Autodesk Inventor part; units mm, degrees
ref_plane "YZ Plane" through (0, 0, 0) normal (1, 0, 0) x (0, 1, 0)
ref_plane "XZ Plane" through (0, 0, 0) normal (0, 1, 0) x (-1, 0, 0)
ref_plane "XY Plane" through (0, 0, 0) normal (0, 0, 1) x (1, 0, 0)
sketch "Sketch1" plane through (0, 0, 0) normal (0, 0, 1) x (1, 0, 0)
  line L0 (0, 0) -> (-9.5, 0)
  line L1 (-9.5, 0) -> (-9.5, 110)
  line L2 (-9.5, 110) -> (-5.5705, 200)
  line L3 (-5.5705, 200) -> (-9, 228)
  line L4 (-9, 228) -> (-9, 232)
  line L5 (-9, 232) -> (-5, 232)
  line L6 (-5, 232) -> (-5, 235)
  line L7 (-5, 235) -> (-6, 235.5774)
  line L8 (-6, 235.5774) -> (-6, 250)
  line L9 (-6, 250) -> (0, 250)
  line L10 (0, 250) -> (0, 0)
  line L11 (0, -50) -> (0, 300)
  line L12 (-11.4, 0) -> (1.9, 0)
  dimension "d0" = 250
  dimension "d1" = 19
  dimension "d2" = 110
  dimension "d5" = 11.141
  dimension "d6" = 12
  dimension "d7" = 3
  dimension "d9" = 18
  dimension "d10" = 4
  dimension "d11" = 10
  dimension "d12" = 60
  dimension "d13" = 18
  dimension "d14" = 2.5
  dimension "d16" = 6.983
  dimension "d17" = 200
  dimension "d18" = 232
  dimension "d19" = 50
  dimension "d20" = 14.4227
revolve "Revolution1" add sketch "Sketch1" angle 360 about axis through (0, -10, 0) along (0, 1, 0)
thread "Thread1"
sketch "Sketch2" plane through (0, 0, 0) normal (0, -1, 0) x (1, 0, 0)
  circle A0 centre (0, 0) radius 9.5
hole "Hole1" at (0, 0, 0) direction (0, 1, 0) diameter 15 depth 80 tip angle 118
chamfer "Chamfer2" distance 2 angle 45 1 edges at (6, 250, 0)
chamfer "Chamfer3" distance 0.5 angle 45 1 edges at (0, 0, 7.5)
chamfer "Chamfer4" distance 1 angle 45 1 edges at (9.5, 0, 0)
properties part number "HM1-001" material "Steel, Alloy"
Part model, mm, in its own coordinate system. A direction names the side the tool comes from. Give positions to 0.01 mm unless a question says otherwise; leave off trailing zeros. Loops run counter-clockwise (first coordinate to the right, second up) from the corner with the lowest first, then second, coordinate; pieces in that order, holes last. Notation, with made-up numbers: (82, -11) -> (89, -11) arc R9 cw to (89, -1) -> close; hole circle Ø5 at (50.5, 19.5). An arc over 180 degrees is marked (long way). Write each question's results on one line, items separated by ' | '. Start each with the question number.
Q1. Band-saw the part on A-A on y = 97. List the corners of the cut face in (x, z).
Q2. Pin check, flat tips, straight feed: P1, Ø1, axis at y = 77.5, z = 6.5, coming from the -X side; P2, Ø6, axis at y = 41.5, z = 5.5, coming from the -X side; P3, Ø8, axis at y = 100, z = 2.5, coming from the +X side; P4, Ø6, axis at y = 142.5, z = -5, coming from the +X side. Stop position of each tip, or through.
Q3. Pull direction Y, two halves, no side cores. Call faces 1 (the face through (1.585, 214.196, -7.135)), 2 (the face through (-3.935, 249.875, -1.239)), 3 (the face through (1.172, 230.028, 8.923)): +Y half, -Y half, draft (parallel to the pull), parting line (faces both ways), or undercut.
Q4. Wall check: L1, parallel to Z at x = 0, y = 31; L2, parallel to X at y = 44, z = -1.75; L3, parallel to Z at x = 5.25, y = 76. Give the ranges that are in metal, low to high.
Q5. Which spindle directions (+Z, -Z, +X, -X, +Y, -Y) get a long thin tool onto all of the face, cutting with end or side? Do faces 4 (the face through (-0.33, 40.806, 7.493)), 5 (the face through (0, 250, 0)), 6 (the face through (6, 242, 0)), 7 (the face through (1.08, 233.52, -4.88)), 8 (the face through (-4.38, 56.26, -8.43)). Say none if no direction does.
Q6. Band-saw the part on B-B on y = 194.5. List the corners of the cut face in (x, z), plus the area to 3 significant figures.
Results are:
1) outline: circle Ø19 at (0, 0)
2) P1: stops at x = -7.37 | P2: stops at x = -9.17 | P3: stops at x = 9.5 | P4: stops at x = 7.84
3) face 1: undercut | face 2: +Y half | face 3: draft
4) L1: z = -9.5 to -7.5, 7.5 to 9.5 | L2: x = -9.34 to -7.29, 7.29 to 9.34 | L3: z = -7.92 to -5.36, 5.36 to 7.92
5) face 4: -Y | face 5: +Z, -Z, +X, -X, +Y | face 6: +Y | face 7: none | face 8: +Y, -Y
6) outline: circle Ø11.62 at (0, 0) | area: 106 mm²
